Geometry: final body of the model. Coordinates: model frame, mm. Face numbers are marked on the shaded views. A direction names the side the tool comes from. Give positions to 0.01 mm unless a question says otherwise; leave off trailing zeros. Order: outer loops, then holes, each group sorted by start corner. A loop starts at its lowest first (then second) coordinate and runs counter-clockwise, first axis right, second up. Notation, with made-up numbers: (9.5, -27.75) -> (58.5, -27.75) arc R19 ccw to (58.5, -16.75) -> close; hole circle Ø6 at (25, 24). An arc over 180 degrees is marked (long way). Answer in a Markdown table with one row per item. Add a question column.
Q1. Cut plane C-C on z = -3.5. Return the cut outline in (x, y).
Q2. Line query: line 1 along X through (y, z) = (1.3, 0); line 2 along X through (y, z) = (4.4, 0). Output: solid intervals per line, ascending. Write a range as from..to.
Q3. Set-up query: the marked faces 4 and 5. Return all of +Z, -Z, +X, -X, +Y, -Y with unobstructed straight access to the full face (end or side cutting, diameter ignored); none if empty.
Q4. Pull-direction query (Z, two-part tool) for the marked faces 1, 2 and 3; classes: +Z half, -Z half, draft (parallel to the pull), parting line (faces both ways), or undercut.
Q5. Cut plane A-A on x = -14. Return the cut outline in (y, z).
Q6. Contact query for flat-ended pins moving along their axis: P1, Ø2, axis at y = 2.5, z = -6.5, coming from the +X side; P2, Ø7, axis at x = 2, z = 1, coming from the -Y side; P3, Ø3, axis at y = 2.5, z = 0.5, coming from the -X side. Output: stop coordinate, or through.
Q7. Cut plane D-D on y = 4.75. Return the cut outline in (x, z).
Q8. Cut plane B-B on z = 0. Return the cut outline in (x, y).
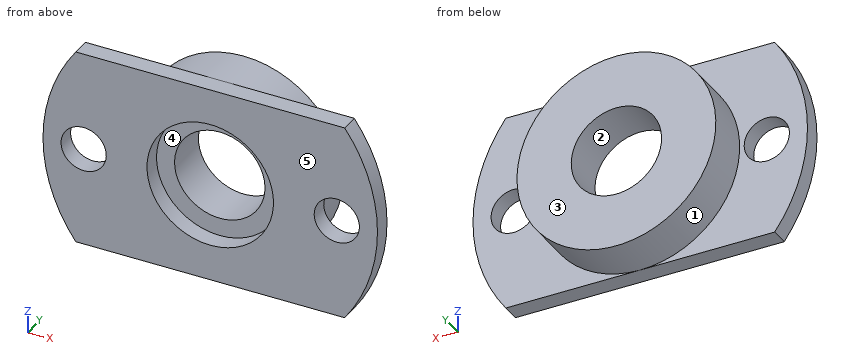
from build123d import *

# Parameters (mm, degrees)
SKETCH_1_R          = 5
EXTRUDE_1_DEPTH     = 2
SKETCH_2_R          = 11
SKETCH_2_R_2        = 5
EXTRUDE_2_DEPTH     = 5
SKETCH_3_R          = 2.5
CUT_EXTRUDE_1_DEPTH = 23.632940596
SKETCH_4_R          = 7
CUT_EXTRUDE_2_DEPTH = 2


with BuildPart() as part:
    # 草图1 → 凸台-拉伸1 (new body)
    with BuildSketch(Plane(origin=(0, 0, 0), x_dir=(1, 0, 0), z_dir=(0, 1, 0))):
        with BuildLine():
            Line((-14.874474781, 11), (14.874474781, 11))
            ThreePointArc((14.874474781, 11), (18.5, 0), (14.874474781, -11))
            Line((14.874474781, -11), (-14.874474781, -11))
            ThreePointArc((-14.874474781, -11), (-18.5, 0), (-14.874474781, 11))
        make_face()
        with Locations(Location((0, 0, 0), (0, 0, 270))):
            Circle(SKETCH_1_R, mode=Mode.SUBTRACT)
    extrude(amount=EXTRUDE_1_DEPTH)

    # 草图2 → 凸台-拉伸2 (add)
    with BuildSketch(Plane(origin=(0, 2, 0), x_dir=(1, 0, 0), z_dir=(0, 1, 0))):
        with Locations(Location((0, 0, 0), (0, 0, 270))):
            Circle(SKETCH_2_R)
        with Locations(Location((0, 0, 0), (0, 0, 270))):
            Circle(SKETCH_2_R_2, mode=Mode.SUBTRACT)
    extrude(amount=EXTRUDE_2_DEPTH)

    # 草图3 → 切除-拉伸1 (cut, through all)
    with BuildSketch(Plane.XZ):
        with Locations(Location((-14, 0, 0), (0, 0, 270))):
            Circle(SKETCH_3_R)
        with Locations(Location((14, 0, 0), (0, 0, 270))):
            Circle(SKETCH_3_R)
    extrude(amount=-CUT_EXTRUDE_1_DEPTH, mode=Mode.SUBTRACT)

    # 草图4 → 切除-拉伸2 (cut)
    with BuildSketch(Plane.XZ):
        with Locations(Location((0, 0, 0), (0, 0, 270))):
            Circle(SKETCH_4_R)
    extrude(amount=-CUT_EXTRUDE_2_DEPTH, mode=Mode.SUBTRACT)


solid = part.part
Completed:
| question | item | result |
|---|---|---|
| 1 | outline | (-18.17, 0) -> (-6.06, 0) -> (-6.06, 2) -> (-3.57, 2) -> (-3.57, 7) -> (-10.43, 7) -> (-10.43, 2) -> (-18.17, 2) -> close; (3.57, 2) -> (6.06, 2) -> (6.06, 0) -> (18.17, 0) -> (18.17, 2) -> (10.43, 2) -> (10.43, 7) -> (3.57, 7) -> close |
| 2 | line 1 | x = -18.5..-16.5, -11.5..-7, 7..11.5, 16.5..18.5 |
| 2 | line 2 | x = -11..-5, 5..11 |
| 3 | face 4 | -Y |
| 3 | face 5 | +Z, -Z, +X, -X, -Y |
| 4 | face 1 | parting line |
| 4 | face 2 | undercut |
| 4 | face 3 | draft |
| 5 | outline | (0, -11) -> (2, -11) -> (2, -2.5) -> (0, -2.5) -> close; (0, 2.5) -> (2, 2.5) -> (2, 11) -> (0, 11) -> close |
| 6 | P1 | stops at x = 17.62 |
| 6 | P2 | stops at y = 2 |
| 6 | P3 | stops at x = -18.5 |
| 7 | outline | circle Ø22 at (0, 0); hole circle Ø10 at (0, 0) |
| 8 | outline | (-18.5, 0) -> (-16.5, 0) -> (-16.5, 2) -> (-18.5, 2) -> close; (-11.5, 0) -> (-7, 0) -> (-7, 2) -> (-5, 2) -> (-5, 7) -> (-11, 7) -> (-11, 2) -> (-11.5, 2) -> close; (5, 2) -> (7, 2) -> (7, 0) -> (11.5, 0) -> (11.5, 2) -> (11, 2) -> (11, 7) -> (5, 7) -> close; (16.5, 0) -> (18.5, 0) -> (18.5, 2) -> (16.5, 2) -> close |
